Verification items for the finished model (mm, model axes). Round coordinates to 2 decimals unless told otherwise and drop trailing zeros. Write each loop counter-clockwise with the first axis right and the second up, starting at its lowest first coordinate (ties: lowest second). Pieces come first, ordered by that corner, then holes. Notation, with made-up numbers: (13, 66.25) - (37, 66.25) arc R10 cw to (37, 77.25) - close; hole circle Ø6 at (-31.5, -35). An arc over 180 degrees is marked (long way). Answer as a JSON object with one key per item and string values.
```python
from build123d import *

# Parameters (mm, degrees)
F0_R     = 10
F1_DEPTH = 10
F2_R     = 5
F3_R     = 20
F4_R     = 10
F5_R     = 10


with BuildPart() as f1:
    # F0 (on Top) → F1 (new body)
    with BuildSketch(Plane.XY):
        with BuildLine():
            ThreePointArc((0, 62.217039), (6.753539, 59.93746), (13.558537, 57.816427))
            ThreePointArc((13.558537, 57.816427), (6.903144, 60.3984), (0, 62.217039))
        make_face()
        with BuildLine():
            ThreePointArc((50.8, 49.186888), (32.043845, 52.917227), (13.558537, 57.816427))
            ThreePointArc((13.558537, 57.816427), (6.753539, 59.93746), (0, 62.217039))
            ThreePointArc((0, 62.217039), (-76.2, 0), (0, -62.217039))
            ThreePointArc((0, -62.217039), (6.753539, -59.93746), (13.558537, -57.816427))
            ThreePointArc((13.558537, -57.816427), (32.043845, -52.917227), (50.8, -49.186888))
            ThreePointArc((50.8, -49.186888), (92.38062, -41.791743), (114.0001, -5.5118))
            ThreePointArc((114.0001, -5.5118), (114.3, 0), (114.0001, 5.5118))
            ThreePointArc((114.0001, 5.5118), (92.38062, 41.791743), (50.8, 49.186888))
        make_face()
        with Locations((-51.278312, 0)):
            Circle(F0_R, mode=Mode.SUBTRACT)
        with BuildLine():
            ThreePointArc((13.558537, -57.816427), (6.753539, -59.93746), (0, -62.217039))
            ThreePointArc((0, -62.217039), (6.903144, -60.3984), (13.558537, -57.816427))
        make_face()
        with BuildLine():
            Line((279.4, 5.5118), (114.0001, 5.5118))
            ThreePointArc((114.0001, 5.5118), (114.3, 0), (114.0001, -5.5118))
            Line((114.0001, -5.5118), (279.4, -5.5118))
            Line((279.4, -5.5118), (279.4, 0))
            Line((279.4, 0), (279.4, 5.5118))
        make_face()
        Polygon((279.4, 18.2118), (279.4, 5.5118), (279.4, 0), (279.4, -5.5118), (279.4, -18.2118), (317.5, -18.2118), (317.5, 18.2118), align=None)
    extrude(amount=F1_DEPTH)

    # F2
    f2_edges = [f1.edges().sort_by_distance(p)[0] for p in [
        (13.558537, 57.816427, 5),
    ]]
    fillet(f2_edges, radius=F2_R)

    # F3
    f3_edges = [f1.edges().sort_by_distance(p)[0] for p in [
        (50.8, 49.186888, 5),
    ]]
    fillet(f3_edges, radius=F3_R)

    # F4
    f4_edges = [f1.edges().sort_by_distance(p)[0] for p in [
        (317.5, 18.2118, 5),
        (279.4, 18.2118, 5),
    ]]
    fillet(f4_edges, radius=F4_R)

    # F5
    f5_edges = [f1.edges().sort_by_distance(p)[0] for p in [
        (317.5, -18.2118, 5),
        (279.4, -18.2118, 5),
    ]]
    fillet(f5_edges, radius=F5_R)


solid = f1.part
```
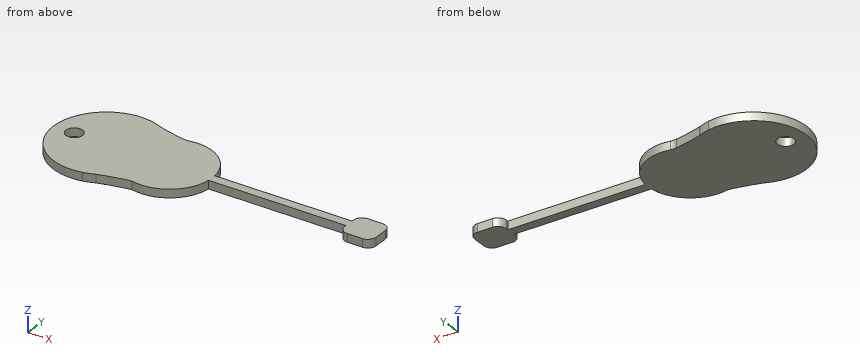
Q1. Section check C-C, the plane y = -23.5. Record the cut outline in (x, z).
Geometry check:
{"outline": "(-71.69, 0) - (108.54, 0) - (108.54, 10) - (-71.69, 10) - close"}
Q2. Material ranges on line 1 along Y through (x, z) = (154, 8); line 2 along X through (y, z) = (-12, 3.5); line 3 along Y through (x, z) = (295.5, 4), recorded low to high. Write a range as [from, to].
Geometry check:
{"line 1": "y = [-5.51, 5.51]", "line 2": "x = [-75.06, 112.86], [280.15, 316.75]", "line 3": "y = [-18.21, 18.21]"}
Q3. Gauge pin test, flat ends, axial feed: P1, Ø0.8, axis at y = 7, z = 5, coming from the -X side; P2, Ø3, axis at x = 185, z = 3.5, coming from the -Y side; P3, Ø3, axis at x = 295.5, z = 7, coming from the -Y side. Record the tip position at first contact, or that the pin passes through.
Geometry check:
{"P1": "stops at x = -75.86", "P2": "stops at y = -5.51", "P3": "stops at y = -18.21"}
Q4. Section check B-B, the plane x = 194.5. Record the cut outline in (y, z), then the cut area to 3 significant figures.
Geometry check:
{"outline": "(-5.51, 0) - (5.51, 0) - (5.51, 10) - (-5.51, 10) - close", "area": "110 mm2"}
Q5. Section check A-A, the plane y = 0. Record the cut outline in (x, z).
Geometry check:
{"outline": "(-76.2, 0) - (-61.28, 0) - (-61.28, 10) - (-76.2, 10) - close; (-41.28, 0) - (317.5, 0) - (317.5, 10) - (-41.28, 10) - close"}
